Autodesk Inventor part; units mm, degrees
ref_plane "YZ Plane" through (0, 0, 0) normal (1, 0, 0) x (0, 1, 0)
ref_plane "XZ Plane" through (0, 0, 0) normal (0, 1, 0) x (-1, 0, 0)
ref_plane "XY Plane" through (0, 0, 0) normal (0, 0, 1) x (1, 0, 0)
sketch "Sketch1" plane through (0, 0, 0) normal (0, 0, 1) x (1, 0, 0)
  line L0 (190.5, 46.6079) -> (218.1822, 46.6079)
  line L1 (218.1822, 46.6079) -> (355.6, 363.7258)
  line L2 (355.6, 363.7258) -> (355.6, 427.6079)
  line L3 (355.6, 427.6079) -> (190.5, 46.6079)
  line L4 (218.1822, 46.6079) -> (355.6, 46.6079) construction
  line L5 (355.6, 46.6079) -> (355.6, 363.7258) construction
  point P0 (0, 0)
  dimension "d0" = 381
  dimension "d2" = 25.4
  dimension "d3" = 165.1
extrude "Extrusion1" add sketch "Sketch1" along normal blind 25.4
shell "Shell1" thickness 1.5875 removed faces 2 at (355.6, 385.0199, 8.4667) at (199.7274, 46.6079, 8.4667)
properties part number "Frame_MainVerticalAngleSupport" material "Aluminum-6061"
Geometry: final body of the model. Coordinates: model frame, mm. A direction names the side the tool comes from. Round coordinates to 2 decimals unless told otherwise and drop trailing zeros. Order: outer loops, then holes, each group sorted by start corner. A loop starts at its lowest first (then second) coordinate and runs counter-clockwise, first axis right, second up. Notation, with made-up numbers: (19, 58) -> (66, 58) arc R13 cw to (66, 74) -> close; hole circle Ø7 at (-29.75, 82). An arc over 180 degrees is marked (long way). Use one line per item in the form item = value. Start each with the question number.
1. Pin query (flat end, axial travel): pin 1 Ø2 at (y, z) = (306.5, 16) entering from +X; pin 2 Ø3 at (x, z) = (256.5, 8.5) entering from -Y; pin 3 Ø8 at (y, z) = (213, 22) entering from -X. Return the tip coordinate at first contact, or that it passes through.
2. Line query: probe 1 along Z at (x, y) = (260, 166.5); probe 2 along X at (y, z) = (226, 21.75); probe 3 along X at (y, z) = (135.5, 10.5). Output: solid intervals per line, ascending.
3. Reachability of faces 4 (the face through (285, 224, 25.4)), 5 (the face through (275.06, 237.75, 12.54)) from +Z, -Z, +X, -X, +Y, -Y: full face, straight path, thin tool, end or side. Return the list, or none.
4. Cut plane C-C (x = 281). Return the cut outline in (y, z), then the cut area to 3 significant figures.
5. Cut plane B-B (y = 211). Return the cut outline in (x, z).
6. Draft query along Y for faces 1 (the face through (286, 222, 1.588)), 2 (the face through (274.206, 239.775, 12.522)), 3 (the face through (285.93, 202.95, 12.52)). Return one class per face: pulls with the +Y half, pulls with the -Y half, needs draft (parallel to the pull), parting line crosses it, or undercut.
7. Cut plane A-A (z = 6). Return the cut outline in (x, y), then the cut area to 3 significant figures.
Solution:
q1.pin_1 = 331.24
q1.pin_2 = 131.57
q1.pin_3 = 260.87
q2.probe_1 = 0 to 1.59, 23.81 to 25.4
q2.probe_2 = 268.24 to 269.97, 294.19 to 295.92
q2.probe_3 = 229.02 to 230.75, 254.97 to 256.7
q3.face_4 = +Z, +X, -X, +Y, -Y
q3.face_5 = none
q4.outline = (191.57, 0) -> (255.45, 0) -> (255.45, 25.4) -> (191.57, 25.4) -> close; hole (195.56, 1.59) -> (251.46, 1.59) -> (251.46, 23.81) -> (195.56, 23.81) -> close
q4.area = 380 mm^2
q5.outline = (261.74, 0) -> (289.42, 0) -> (289.42, 25.4) -> (261.74, 25.4) -> close; hole (263.47, 1.59) -> (287.69, 1.59) -> (287.69, 23.81) -> (263.47, 23.81) -> close
q6.face_1 = undercut
q6.face_2 = pulls with the +Y half
q6.face_3 = pulls with the -Y half
q7.outline = (190.5, 46.61) -> (192.23, 46.61) -> (355.6, 423.62) -> (355.6, 427.61) -> close; (216.45, 46.61) -> (218.18, 46.61) -> (355.6, 363.73) -> (355.6, 367.72) -> close
q7.area = 1,210 mm^2
